Read the model definition and answer for the solid it produces. Units are mm, in the model's axes. A direction names the side the tool comes from. Round coordinates to 2 decimals unless told otherwise and drop trailing zeros. Order: outer loops, then holes, each group sorted by start corner. A loop starts at its lowest first (then second) coordinate and runs counter-clockwise, first axis right, second up. Notation, with made-up numbers: M -30.5,-18.5 L 2.5,-18.5 A31 ccw 2.5,20.5 Z; hole C 24,53.5 d6. An arc over 180 degrees is marked long. Answer as CSV lines item,"result".
```python
from build123d import *

# Parameters (mm, degrees)
F1_DEPTH      = 10
F1_DEPTH_BACK = 10
F2_DEPTH      = 1.5
F2_DEPTH_BACK = 1.5
F3_R          = 2
F4_DEPTH      = 5
F4_DEPTH_BACK = 5


with BuildPart() as f1:
    # F0 (on Front) → F1 (new body, two sides)
    with BuildSketch(Plane.XZ) as f1_sk:
        Polygon((25.327755, 0), (17.327755, 0), (5.327755, 0), (-2.672245, 0), (-2.672245, -4), (25.327755, -4), align=None)
    extrude(amount=F1_DEPTH)
    extrude(f1_sk.sketch, amount=-F1_DEPTH_BACK)

    # F0 (on Front) → F2 (join, two sides)
    with BuildSketch(Plane.XZ) as f2_sk:
        with BuildLine():
            Line((5.327755, 0), (17.327755, 0))
            Line((17.327755, 0), (17.327755, 12))
            ThreePointArc((17.327755, 12), (11.327755, 6), (5.327755, 12))
            Line((5.327755, 12), (5.327755, 0))
        make_face()
        with BuildLine():
            ThreePointArc((5.327755, 12), (11.327755, 6), (17.327755, 12))
            Line((17.327755, 12), (13.327755, 12))
            ThreePointArc((13.327755, 12), (11.327755, 10), (9.327755, 12))
            Line((9.327755, 12), (5.327755, 12))
        make_face()
        with BuildLine():
            Line((13.327755, 12), (17.327755, 12))
            ThreePointArc((17.327755, 12), (11.327755, 18), (5.327755, 12))
            Line((5.327755, 12), (9.327755, 12))
            ThreePointArc((9.327755, 12), (11.327755, 14), (13.327755, 12))
        make_face()
    extrude(amount=F2_DEPTH)
    extrude(f2_sk.sketch, amount=-F2_DEPTH_BACK)

    # F3 (on face) → F4 (cut, two sides)
    with BuildSketch(Plane.XY) as f4_sk:
        with Locations((1.327755, 0)):
            Circle(F3_R)
        with Locations((21.327755, 0)):
            Circle(F3_R)
    extrude(amount=-F4_DEPTH, mode=Mode.SUBTRACT)
    extrude(f4_sk.sketch, amount=-F4_DEPTH_BACK, mode=Mode.SUBTRACT)


solid = f1.part
```
Item 1: Find the intervals of material crossed by probe 1 along X at (y, z) = (0, 3.25); probe 2 along Z at (x, y) = (12, -5); probe 3 along Y at (x, z) = (16.25, 15), in increasing order. Write a range as [from, to].
Ans:
probe 1,"[5.33, 17.33]"
probe 2,"[-4, 0]"
probe 3,"[-1.5, 1.5]"
Item 2: A tool of negligible diameter and unlimited length cuts with its end or side. For faces 4 (the face through (0.89, -1.95, -1.97)), 5 (the face through (17.328, 0, 6)), 6 (the face through (25.328, 0, -2)), 7 (the face through (11, 1.5, 9)), 8 (the face through (11, -1.5, 9)), from which of +Z, -Z, +X, -X, +Y, -Y can it reach the whole face along a straight path? Write none if from no direction.
Ans:
face 4,"+Z, -Z"
face 5,"+Z, +X, +Y, -Y"
face 6,"+Z, -Z, +X, +Y, -Y"
face 7,"+Z, +X, -X, +Y"
face 8,"+Z, +X, -X, -Y"
Item 3: A cutting plane is placed at A-A, the plane y = 0. Determine the outline of the cut face in (x, z).
Ans:
outline,"M -2.67,-4 L -0.67,-4 L -0.67,0 L -2.67,0 Z; M 3.33,-4 L 19.33,-4 L 19.33,0 L 17.33,0 L 17.33,12 A6 ccw 5.33,12 L 5.33,0 L 3.33,0 Z; M 23.33,-4 L 25.33,-4 L 25.33,0 L 23.33,0 Z; hole C 11.33,12 d4"
Item 4: A cutting plane is placed at B-B, the plane x = 11.5. Determine the outline of the cut face in (y, z), and give its area (3 significant figures).
Ans:
outline,"M -10,-4 L 10,-4 L 10,0 L 1.5,0 L 1.5,10.01 L -1.5,10.01 L -1.5,0 L -10,0 Z; M -1.5,13.99 L 1.5,13.99 L 1.5,18 L -1.5,18 Z"
area,"122 mm2"
Item 5: Determine the mould class of faces 1 (the face through (11, -10, -2)), 2 (the face through (5.328, 0, 6)), 3 (the face through (23.175, -0.766, -1.972)) for opening direction Y: +Y half, -Y half, draft (parallel to the pull), parting line (faces both ways), or undercut.
Ans:
face 1,"-Y half"
face 2,"draft"
face 3,"undercut"
Item 6: Flat-ended cylindrical pins translate along their axes: pin 1 (8 mm diameter, centred on x = 6, z = 8, fed in from +Y); pin 2 (1.5 mm diameter, centred on y = -0.5, z = 8, fed in from +X); pin 3 (4 mm diameter, centred on x = 13.5, y = -5.5, fed in from +Z); pin 4 (2.5 mm diameter, centred on x = 21.33, y = 0, fed in from -Z). Find the tip coordinate at first contact, or state that the pin passes through.
Ans:
pin 1,"y = 1.5"
pin 2,"x = 17.33"
pin 3,"z = 0"
pin 4,"through"
Item 7: A cutting plane is placed at C-C, the plane x = 6.5. Determine the outline of the cut face in (y, z).
Ans:
outline,"M -10,-4 L 10,-4 L 10,0 L 1.5,0 L 1.5,15.56 L -1.5,15.56 L -1.5,0 L -10,0 Z"
Item 8: A cutting plane is placed at D-D, the plane y = -6.5. Determine the outline of the cut face in (x, z).
Ans:
outline,"M -2.67,-4 L 25.33,-4 L 25.33,0 L -2.67,0 Z"
